The model under review builds one solid part; all positions refer to its coordinate system, in mm. Face numbers are marked on the shaded views. A direction names the side the tool comes from. Give positions to 0.01 mm unless a question says otherwise; leave off trailing zeros. Order: outer loops, then holes, each group sorted by start corner. A loop starts at its lowest first (then second) coordinate and runs counter-clockwise, first axis right, second up.
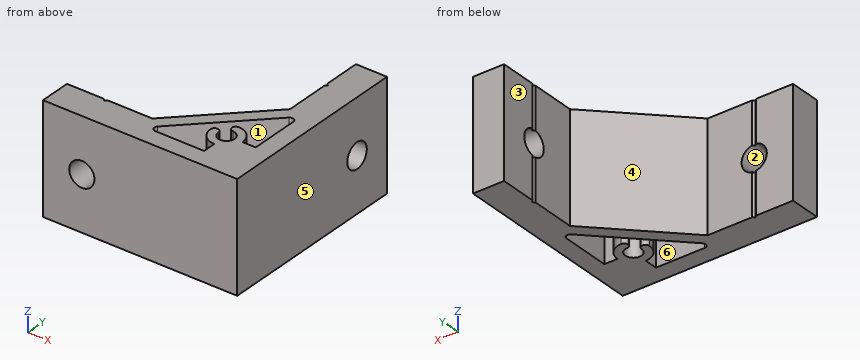
```python
from build123d import *

# Parameters (mm, degrees)
EXTRUDE_1_DEPTH     = 14
SKETCH_2_R          = 3.25
CUT_EXTRUDE_1_DEPTH = 9
SKETCH_3_R          = 3.25
CUT_EXTRUDE_2_DEPTH = 9


with BuildPart() as part:
    # Эскиз1 → Бобышка-Вытянуть1 (new body, symmetric)
    with BuildSketch(Plane.XY):
        Polygon((-50, 0), (0, 0), (0, 50), (-8, 50), (-8, 40.5), (-7.5, 40), (-8, 39.5), (-8, 28), (-28, 8), (-39.5, 8), (-40, 7.5), (-40.5, 8), (-50, 8), align=None)
        with BuildLine():
            Line((-4.5, 12), (-4.5, 24.560303038))
            ThreePointArc((-4.5, 24.560303038), (-5.117316568, 25.484182571), (-6.207106781, 25.267409819))
            Line((-6.207106781, 25.267409819), (-25.267409819, 6.207106781))
            ThreePointArc((-25.267409819, 6.207106781), (-25.484182571, 5.117316568), (-24.560303038, 4.5))
            Line((-24.560303038, 4.5), (-12, 4.5))
            Line((-12, 4.5), (-12, 7.9))
            ThreePointArc((-12, 7.9), (-14.899137803, 9.100862197), (-16.1, 12))
            ThreePointArc((-16.1, 12), (-15.1, 13), (-14.1, 12))
            ThreePointArc((-14.1, 12), (-10.51507576, 10.51507576), (-12, 14.1))
            ThreePointArc((-12, 14.1), (-13, 15.1), (-12, 16.1))
            ThreePointArc((-12, 16.1), (-9.100862197, 14.899137803), (-7.9, 12))
            Line((-7.9, 12), (-4.5, 12))
        make_face(mode=Mode.SUBTRACT)
    extrude(amount=EXTRUDE_1_DEPTH, both=True)

    # Эскиз2 → Вырез-Вытянуть1 (cut, through all)
    with BuildSketch(Plane.ZY.offset(8)):
        with Locations(Location((0, 40, 0), (0, 0, 270))):  # turned: the seam where the file's is
            Circle(SKETCH_2_R)
    extrude(amount=-CUT_EXTRUDE_1_DEPTH, mode=Mode.SUBTRACT)

    # Эскиз3 → Вырез-Вытянуть2 (cut, through all)
    with BuildSketch(Plane(origin=(0, 8, 0), x_dir=(1, 0, 0), z_dir=(0, 1, 0))):
        with Locations(Location((-40, 0, 0), (0, 0, 180))):  # turned: the seam where the file's is
            Circle(SKETCH_3_R)
    extrude(amount=-CUT_EXTRUDE_2_DEPTH, mode=Mode.SUBTRACT)


solid = part.part
```
1. Draft analysis for pull direction X (two halves, no side actions). For the marked faces 4, 5 and 6, state which applies: pulls with the +X half, pulls with the -X half, needs draft (parallel to the pull), parting line crosses it, or undercut.
2. Take a section at D-D (y = 33). Write out the cut boundary in (x, z).
3. Take a section at B-B (x = -18). Write out the cut boundary in (y, z), and give its area (3 significant figures).
4. To check wall thickness, follow line 1 (X direction, y = 3, z = 0); line 2 (X direction, y = 7.5, z = -1); line 3 (Z direction, x = -40, y = 5.25). State the ranges of each line that lie inside material, in increasing order.
5. Take a section at C-C (y = 15.1). Write out the cut boundary in (x, z).
6. For the marked faces 1, 2 and 3, list the 3-axis set-ups (+Z, -Z, +X, -X, +Y, -Y) from which the entire face can be reached by the end or side of a thin tool; tool diameter is ignored.
7. Insertion check: pin 1 (12.5 mm diameter, centred on x = -34, z = 2.5, fed in from +Y); pin 2 (4 mm diameter, centred on x = -17.5, z = 2.5, fed in from +Y); pin 3 (10 mm diameter, centred on x = -28.5, z = -0.5, fed in from +Y). Each pin has a flat end and moves straight along its axis. Give the tip position at first contact, or say it passes through.
8. Take a section at A-A (z = 0). Write out the cut boundary in (x, y).
Answer:
1. face 4: pulls with the -X half
1. face 5: pulls with the +X half
1. face 6: undercut
2. outline: (-8, -14) - (0, -14) - (0, 14) - (-8, 14) - close
3. outline: (0, -14) - (4.5, -14) - (4.5, 14) - (0, 14) - close; (13.47, -14) - (18, -14) - (18, 14) - (13.47, 14) - close
3. area: 253 mm2
4. line 1: x = -50 to -43.25, -36.75 to 0
4. line 2: x = -50 to -43.09, -36.91 to -23.97, -12 to 0
4. line 3: z = -14 to -3.25, 3.25 to 14
5. outline: (-20.9, -14) - (-16.37, -14) - (-16.37, 14) - (-20.9, 14) - close; (-13, -14) - (-9.32, -14) - (-9.32, 14) - (-13, 14) - close; (-4.5, -14) - (0, -14) - (0, 14) - (-4.5, 14) - close
6. face 1: +Z, -Z
6. face 2: +Y, -Y
6. face 3: +Z, -Z, -X, +Y
7. pin 1: stops at y = 8.25
7. pin 2: stops at y = 20.5
7. pin 3: stops at y = 12.5
8. outline: (-50, 0) - (-43.25, 0) - (-43.25, 8) - (-50, 8) - close; (-36.75, 0) - (0, 0) - (0, 36.75) - (-8, 36.75) - (-8, 28) - (-28, 8) - (-36.75, 8) - close; (-8, 43.25) - (0, 43.25) - (0, 50) - (-8, 50) - close; hole (-25.27, 6.21) arc R1 ccw to (-24.56, 4.5) - (-12, 4.5) - (-12, 7.9) arc R4.1 cw to (-16.1, 12) arc R1 cw to (-14.1, 12) arc R2.1 ccw (long way) to (-12, 14.1) arc R1 cw to (-12, 16.1) arc R4.1 cw to (-7.9, 12) - (-4.5, 12) - (-4.5, 24.56) arc R1 ccw to (-6.21, 25.27) - close
